Could you check a few things on this model? Use its own coordinates, in mm. A direction names the side the tool comes from. Give positions to 0.01 mm unless a question says otherwise; leave off trailing zeros. One line per item, written item: value. Start each with the question number.
Q1. For faces 1 (the face through (-1.08, -4.88, 7.64)), 2 (the face through (0.3, 5.4, 65.3)), which set-ups out of +Z, -Z, +X, -X, +Y, -Y let a thin tool reach every point of the face, with its end or its side?
Q2. If I drill on line 1 (Z direction, x = -14, y = -1); line 2 (Z direction, x = 15, y = 1); line 3 (X direction, y = 0, z = 24), over which ranges is the centre line in solid material (lowest first)? Write a range as from..to.
Q3. I'm going to push flat-ended pins straight in: P1, Ø1.5, axis at y = 9.5, z = -2, coming from the +X side; P2, Ø8, axis at x = -7, y = -22, coming from the -Z side; P3, Ø5, axis at y = -8.5, z = 43, coming from the +X side; P4, Ø6, axis at x = 0, y = 0, coming from the +Z side. Where does each tip first touch, or does it pass through?
```python
from build123d import *

# Parameters (mm, degrees)
F3_W     = 32.0855062455
F3_H     = 31.694107689
F4_DEPTH = 18.5
F5_R     = 5
F6_DEPTH = 172.9


with BuildPart() as f1:
    # F0 (on Front) → F1 (revolve)
    with BuildSketch(Plane.XZ):
        with BuildLine():
            Line((0, 76.1397406459), (0, 74.7660771012))
            Line((0, 74.7660771012), (0, -48.4679415822))
            add(Edge.make_bspline(
                [(0, -48.4679415822), (1.08196968, -50.0808969928), (4.3605942772, -54.9685342168), (24.6603145313, -36.419058951), (26.6652045018, 10.6134220282), (11.7971467763, 25.3826350696), (10.3892143692, 26.3787310574), (6.7118340158, 38.435006696), (10.6774127447, 44.1303949518), (1.721249837, 57.4634062624), (32.0136776372, 62.2713275471), (34.3508236047, 79.0017212819), (2.5772251559, 78.0817526941), (0, 76.1397406459)],
                knots=[0, 0, 0, 0, 0.0529922354, 0.1605790343, 0.3211416148, 0.4177492714, 0.4486271125, 0.5267484863, 0.5879608779, 0.6605030222, 0.7764602024, 0.8454861286, 0.9727080848, 0.9727080848, 0.9727080848, 0.9727080848], degree=3))
        make_face()
    revolve(axis=Axis((0, 0, 15.4695112284), (0, 0, -1)))

    # F3 (on offset) → F4 (cut)
    with BuildSketch(Plane.XY.offset(83.8)):
        with Locations((0.558228232, 1.689506229)):
            Rectangle(F3_W, F3_H)
    extrude(amount=-F4_DEPTH, mode=Mode.SUBTRACT)

    # F5 (on offset) → F6 (cut)
    with BuildSketch(Plane.XY.offset(83.8)):
        Circle(F5_R)
    extrude(amount=-F6_DEPTH, mode=Mode.SUBTRACT)


solid = f1.part
```
Worked answers:
1. face 1: +Z, -Z
1. face 2: +Z
2. line 1: z = -44.36..22.97, 58.54..65.3
2. line 2: z = -43..21.81, 58.96..65.3
2. line 3: x = -13.08..-5, 5..13.08
3. P1: stops at x = 22.45
3. P2: stops at z = -35.82
3. P3: stops at x = 6.71
3. P4: passes through
